Drawing for the job (mm, zero at the part's lowest x, y, z). A direction names the side the tool comes from. Round coordinates to 2 decimals unless told otherwise and drop trailing zeros. Order: outer loops, then holes, each group sorted by start corner. A loop starts at its lowest first (then second) coordinate and runs counter-clockwise, first axis right, second up. Notation, with made-up numbers: M -10.75,-26.5 L 47.25,-26.5 A16 cw 47.25,-21.5 Z; hole C 67.25,62.5 d5. An arc over 180 degrees is marked long. One line per item, written item: value. Start each with the question number.
Item 1: Band-saw the part on C-C, the plane z = 23.5. Write the cut outline in (x, y).
Item 2: Pin check, flat tips, straight feed: pin 1 (6 mm diameter, centred on x = 19.5, z = 24, fed in from +Y); pin 2 (1.5 mm diameter, centred on x = 16.5, y = 7.5, fed in from -Z); pin 3 (4.5 mm diameter, centred on x = 13, y = 11, fed in from +Z). Stop position of each tip, or through.
Item 3: Band-saw the part on B-B, the plane y = 14. Write the cut outline in (x, z).
Item 4: Band-saw the part on D-D, the plane y = 2.25. Write the cut outline in (x, z).
Item 5: Band-saw the part on A-A, the plane x = 13. Write the cut outline in (y, z).
Item 6: Tool access for the marked faces 1 and 2: list every direction of +Z, -Z, +X, -X, +Y, -Y with a clear straight run to the whole face (end or side of a thin tool).
Item 7: Probe L1, parallel to Y at x = 13, z = 24.35; L2, parallel to Y at x = 23, z = 23.25; L3, parallel to X at y = 3.5, z = 21. List the from-to ranges inside material, lowest first.
Item 8: Two-plate mould, pull along Y, no slides. Class the marked faces 3, 4 and 5: +Y half, -Y half, draft (parallel to the pull), parting line (faces both ways), or undercut.
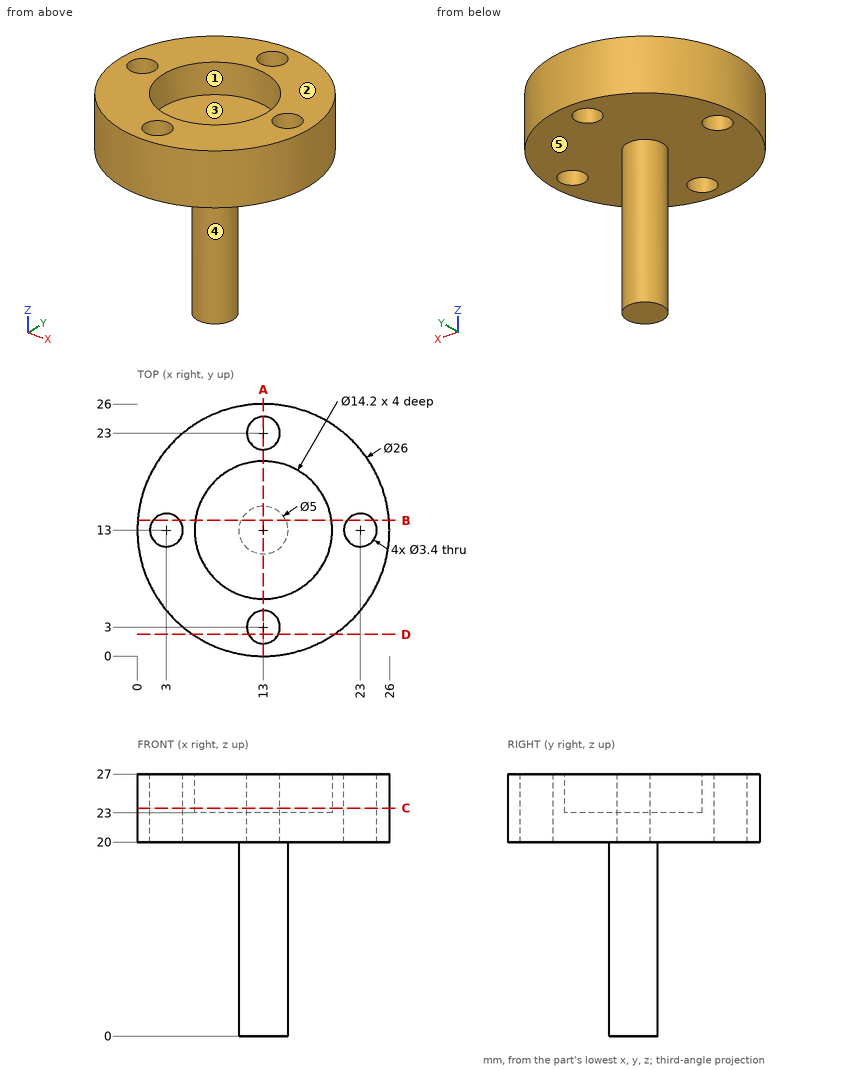
Output:
1. outline: C 13,13 d26; hole C 3,13 d3.4; hole C 13,13 d14.2; hole C 13,3 d3.4; hole C 13,23 d3.4; hole C 23,13 d3.4
2. pin 1: stops at y = 25.52
2. pin 2: stops at z = 20
2. pin 3: stops at z = 23
3. outline: M 0.04,20 L 1.63,20 L 1.63,27 L 0.04,27 Z; M 4.37,20 L 10.71,20 L 10.71,0 L 15.29,0 L 15.29,20 L 21.63,20 L 21.63,27 L 20.03,27 L 20.03,23 L 5.97,23 L 5.97,27 L 4.37,27 Z; M 24.37,20 L 25.96,20 L 25.96,27 L 24.37,27 Z
4. outline: M 5.69,20 L 11.47,20 L 11.47,27 L 5.69,27 Z; M 14.53,20 L 20.31,20 L 20.31,27 L 14.53,27 Z
5. outline: M 0,20 L 1.3,20 L 1.3,27 L 0,27 Z; M 4.7,20 L 10.5,20 L 10.5,0 L 15.5,0 L 15.5,20 L 21.3,20 L 21.3,27 L 20.1,27 L 20.1,23 L 5.9,23 L 5.9,27 L 4.7,27 Z; M 24.7,20 L 26,20 L 26,27 L 24.7,27 Z
6. face 1: +Z
6. face 2: +Z, +X, -X, +Y, -Y
7. L1: y = 0 to 1.3, 4.7 to 5.9, 20.1 to 21.3, 24.7 to 26
7. L2: y = 4.69 to 11.3, 14.7 to 21.31
7. L3: x = 4.13 to 11.38, 14.62 to 21.87
8. face 3: undercut
8. face 4: parting line
8. face 5: draft
